Read the model definition and answer for the solid it produces. Units are mm, in the model's axes. A direction names the side the tool comes from. Round coordinates to 2 decimals unless told otherwise and drop trailing zeros. Write each loop counter-clockwise with the first axis right and the second up, starting at its lowest first coordinate (ties: lowest second). Pieces come first, ordered by that corner, then holes. Notation, with made-up numbers: (11.25, 50.25) - (57.25, 50.25) arc R25 ccw to (57.25, 66.25) - close; hole circle Ø3 at (-4, -24.5). An arc over 180 degrees is marked (long way). Use one line per item in the form item = value. Start each with the question number.
1) The part is cut by section A-A, the plane x = 5. Give the vertices of the cut face in (y, z), plus the area to 3 significant figures.
2) The part is cut by section C-C, the plane x = 90. Give the vertices of the cut face in (y, z), plus the area to 3 significant figures.
3) Each of these flat-tipped pins is pushed along its axis until it touches: pin 1 (8 mm diameter, centred on x = 72.5, y = 22.5, fed in from +Z); pin 2 (4 mm diameter, centred on x = 97, y = -4.5, fed in from +Z); pin 3 (1.5 mm diameter, centred on y = -5, z = 1.5, fed in from +X); pin 4 (3 mm diameter, centred on y = 20.5, z = 4, fed in from -X). Where does it stop, or does it pass through?
4) For faces 4 (the face through (49, 21, 4)), 5 (the face through (49.3, 9.926, 7.896)), 6 (the face through (5, -4, 3)), 7 (the face through (9, -4, 1)), determine the directions among +Z, -Z, +X, -X, +Y, -Y from which every point of the face is accessible in a straight line to the end or side of a thin tool.
5) Consider line 1 along X through (y, z) = (4, 6.5); line 2 along Y through (x, z) = (5, 1.6); line 3 along X through (y, z) = (-6, 1). Determine where each line is inside the solid, lowest interval first. Write a range as from..to.
6) The part is cut by section D-D, the plane y = 12. Give the vertices of the cut face in (x, z).
7) The part is cut by section B-B, the plane x = 42. Give the vertices of the cut face in (y, z).
8) For a pull along X with two mould halves and no side action, classify faces 1 (the face through (1, -3, 1)), 2 (the face through (49, 25, 2)), 3 (the face through (91, -3, 1)) as released by +X, released by -X, zero draft, split by the parting line, or undercut.
from build123d import *

# Parameters (mm, degrees)
SKETCH_1_W          = 100
SKETCH_1_H          = 25
EXTRUDE_1_DEPTH     = 4
SKETCH_2_W          = 100
SKETCH_2_H          = 10.76
EXTRUDE_2_DEPTH     = 10
CUT_EXTRUDE_1_DEPTH = 105.024035684
SKETCH_6_R          = 1.4
CUT_EXTRUDE_2_DEPTH = 102.768128406
SKETCH_7_R          = 1.75
EXTRUDE_3_DEPTH     = 3
SKETCH_8_R          = 1.75
CUT_EXTRUDE_3_DEPTH = 104.561575886


with BuildPart() as part:
    # 스케치1 → 보스-돌출1 (new body)
    with BuildSketch(Plane.XY):
        with Locations((50, 12.5)):
            Rectangle(SKETCH_1_W, SKETCH_1_H)
    extrude(amount=EXTRUDE_1_DEPTH)

    # 스케치2 → 보스-돌출2 (add)
    with BuildSketch(Plane.XY.offset(4)):
        with Locations((50, 5.38)):
            Rectangle(SKETCH_2_W, SKETCH_2_H)
    extrude(amount=EXTRUDE_2_DEPTH)

    # 스케치5 → 컷-돌출1 (cut, through all)
    with BuildSketch(Plane.ZY):
        Polygon((1.96, 10.76), (19, 8.365184177), (4, 17.874325465), align=None)
    extrude(amount=-CUT_EXTRUDE_1_DEPTH, mode=Mode.SUBTRACT)

    # 스케치6 → 컷-돌출2 (cut, through all)
    with BuildSketch(Plane(origin=(0, 10.821712533, 1.520892512), x_dir=(1, 0, 0), z_dir=(0, 0.9902680687415709, 0.1391731009600619))):
        with Locations(Location((16, -5.741746822, 0), (0, 0, 270))):
            Circle(SKETCH_6_R)
        with Locations(Location((84, -5.741746822, 0), (0, 0, 270))):
            Circle(SKETCH_6_R)
    extrude(amount=-CUT_EXTRUDE_2_DEPTH, mode=Mode.SUBTRACT)

    # 스케치7 → 보스-돌출3 (add)
    # profile 1 of 2: a face of its own
    with BuildSketch(Plane(origin=(0, 0, 0), x_dir=(-1, 0, 0), z_dir=(0, 0, -1))):
        with BuildLine():
            Line((-99, -7), (-99, 0))
            Line((-99, 0), (-91, 0))
            Line((-91, 0), (-91, -7))
            ThreePointArc((-91, -7), (-95, -11), (-99, -7))
        make_face()
        with Locations((-95, -7)):
            Circle(SKETCH_7_R, mode=Mode.SUBTRACT)
    # profile 2 of 2: a face of its own
    with BuildSketch(Plane(origin=(0, 0, 0), x_dir=(-1, 0, 0), z_dir=(0, 0, -1))):
        with BuildLine():
            Line((-9, -7), (-9, 0))
            Line((-9, 0), (-1, 0))
            Line((-1, 0), (-1, -7))
            ThreePointArc((-1, -7), (-5, -11), (-9, -7))
        make_face()
        with Locations((-5, -7)):
            Circle(SKETCH_7_R, mode=Mode.SUBTRACT)
    extrude(amount=-EXTRUDE_3_DEPTH)

    # 스케치8 → 컷-돌출3 (cut, through all)
    with BuildSketch(Plane.XY.offset(4)):
        with Locations((10, 21.437162733)):
            Circle(SKETCH_8_R)
        with Locations((90, 21.437162733)):
            Circle(SKETCH_8_R)
    extrude(amount=-CUT_EXTRUDE_3_DEPTH, mode=Mode.SUBTRACT)


solid = part.part
Geometry results:
q1.outline = (-11, 0) - (-8.75, 0) - (-8.75, 3) - (-11, 3) - close; (-5.25, 0) - (25, 0) - (25, 4) - (17.87, 4) - (10.76, 1.96) - (9.07, 14) - (0, 14) - (0, 3) - (-5.25, 3) - close
q1.area = 213 mm2
q2.outline = (0, 0) - (19.69, 0) - (19.69, 4) - (17.87, 4) - (10.76, 1.96) - (9.07, 14) - (0, 14) - close; (23.19, 0) - (25, 0) - (25, 4) - (23.19, 4) - close
q2.area = 176 mm2
q3.pin_1 = 4
q3.pin_2 = 3
q3.pin_3 = 99
q3.pin_4 = 0
q4.face_4 = +Z, +X, -X, +Y
q4.face_5 = +Z, +X, -X
q4.face_6 = +Z, +X, -X, -Y
q4.face_7 = +Z, -Z, -Y
q5.line_1 = 0..14.61, 17.39..82.61, 85.39..100
q5.line_2 = -11..-8.75, -5.25..25
q5.line_3 = 1..3.56, 6.44..9, 91..93.56, 96.44..99
q6.outline = (0, 0) - (100, 0) - (100, 2.32) - (0, 2.32) - close
q7.outline = (0, 0) - (25, 0) - (25, 4) - (17.87, 4) - (10.76, 1.96) - (9.07, 14) - (0, 14) - close
q8.face_1 = released by -X
q8.face_2 = zero draft
q8.face_3 = undercut
